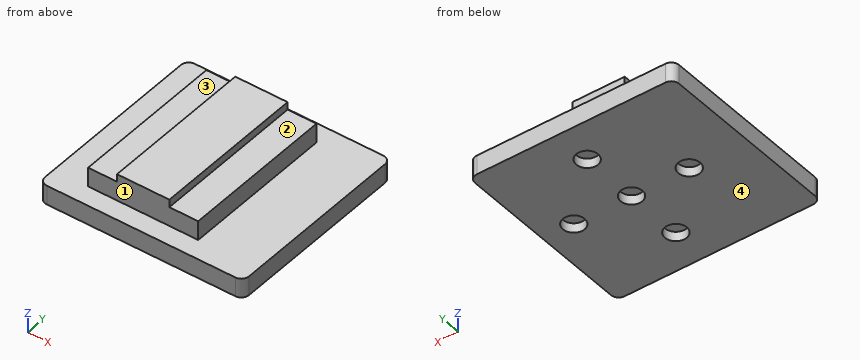
Autodesk Inventor part; units mm, degrees
ref_plane "YZ Plane" through (0, 0, 0) normal (1, 0, 0) x (0, 1, 0)
ref_plane "XZ Plane" through (0, 0, 0) normal (0, 1, 0) x (-1, 0, 0)
ref_plane "XY Plane" through (0, 0, 0) normal (0, 0, 1) x (1, 0, 0)
sketch "Sketch1" plane through (0, 0, 0) normal (0, 0, 1) x (1, 0, 0)
  line L0 (-24.5, 25) -> (24.5, 25)
  line L1 (26.5, 23) -> (26.5, -23)
  line L2 (24.5, -25) -> (-24.5, -25)
  line L3 (-26.5, -23) -> (-26.5, 23)
  arc A0 (-24.5, 25) -> (-26.5, 23) centre (-24.5, 23) ccw
  arc A1 (-26.5, -23) -> (-24.5, -25) centre (-24.5, -23) ccw
  arc A2 (24.5, -25) -> (26.5, -23) centre (24.5, -23) ccw
  arc A3 (26.5, 23) -> (24.5, 25) centre (24.5, 23) ccw
  point P0 (0, 0)
  point P1 (-26.5, 25)
  point P2 (26.5, -25)
  point P3 (26.5, 25)
  dimension "d0" = 53
  dimension "d2" = 2
  dimension "d3" = 25
  dimension "d4" = 50
  dimension "d5" = 26.5
extrude "base" add sketch "Sketch1" along normal blind 5
sketch "Sketch3" plane through (0, 0, 0) normal (0, 0, -1) x (-1, 0, 0)
  line L0 (26.5, 23) -> (26.5, -23)
  circle A0 centre (-3.5, 15) radius 2.825
  circle A1 centre (-18.5, 0) radius 2.825
  circle A2 centre (-3.5, 0) radius 2.825
  circle A3 centre (-3.5, -15) radius 2.825
  circle A4 centre (11.5, 0) radius 2.825
  point P0 (0, 0)
  dimension "d14" = 15
  dimension "d15" = 15
  dimension "d16" = 15
  dimension "d17" = 15
  dimension "d18" = 15
  dimension "d56" = 5.65
  dimension "d57" = 5.65
  dimension "d58" = 5.65
  dimension "d59" = 5.65
  dimension "d60" = 5.65
extrude "magnetExt" cut sketch "Sketch3" against normal blind 2.5
sketch "Sketch7" plane through (0, 0, 5) normal (0, 0, 1) x (1, 0, 0)
  line L0 (-17.6, 20) -> (11, 20)
  line L1 (11, 20) -> (11, -20)
  line L2 (11, -20) -> (-17.6, -20)
  line L3 (-17.6, -20) -> (-17.6, 20)
  line L4 (-26.5, 23) -> (-26.5, -23)
  point P0 (0, 0)
  dimension "d70" = 40
  dimension "d71" = 20
  dimension "d72" = 28.6
  dimension "d73" = 8.9
extrude "spacerOne" add sketch "Sketch7" along normal blind 5
sketch "Sketch8" plane through (0, 0, 10) normal (0, 0, 1) x (1, 0, 0)
  line L0 (-10.1, 20) -> (3.5, 20)
  line L1 (3.5, 20) -> (3.5, -20)
  line L2 (3.5, -20) -> (-10.1, -20)
  line L3 (-10.1, -20) -> (-10.1, 20)
  line L4 (-26.5, 23) -> (-26.5, -23)
  point P0 (0, 0)
  dimension "d76" = 40
  dimension "d77" = 20
  dimension "d78" = 13.6
  dimension "d79" = 30
extrude "sample" add sketch "Sketch8" along normal blind 2
equation "\"d56\" = d60"
equation "\"d57\" = d60"
equation "\"d58\" = d60"
equation "\"d59\" = d60"
equation "\"d1\" = d0"
properties part number "chamberInsertFlat"
Model file for the job. Use its own axes, mm. Face numbers are marked on the shaded views. A direction names the side the tool comes from. Round coordinates to 2 decimals unless told otherwise and drop trailing zeros. Loops run counter-clockwise (first coordinate to the right, second up) from the corner with the lowest first, then second, coordinate; pieces in that order, holes last.
1. Band-saw the part on C-C, the plane y = 0. List the corners of the cut face in (x, z) (3 decimals), and give its area (3 significant figures).
Check values:
outline: (-26.5, 0) - (-14.325, 0) - (-14.325, 2.5) - (-8.675, 2.5) - (-8.675, 0) - (0.675, 0) - (0.675, 2.5) - (6.325, 2.5) - (6.325, 0) - (15.675, 0) - (15.675, 2.5) - (21.325, 2.5) - (21.325, 0) - (26.5, 0) - (26.5, 5) - (11, 5) - (11, 10) - (3.5, 10) - (3.5, 12) - (-10.1, 12) - (-10.1, 10) - (-17.6, 10) - (-17.6, 5) - (-26.5, 5) - close
area: 393 mm2
2. Wall check: probe 1 along Y at (x, z) = (3.5, 0.95) (3 decimals); probe 2 along X at (y, z) = (-2.5, 1.25); probe 3 along Z at (x, y) = (22, 0). Give the ranges that are in metal, low to high.
Check values:
probe 1: y = -25 to -17.825, -12.175 to -2.825, 2.825 to 12.175, 17.825 to 25
probe 2: x = -26.5 to -12.82, -10.18 to 2.18, 4.82 to 17.18, 19.82 to 26.5
probe 3: z = 0 to 5
3. Band-saw the part on A-A, the plane y = -15. List the corners of the cut face in (x, z) (3 decimals).
Check values:
outline: (-26.5, 0) - (0.675, 0) - (0.675, 2.5) - (6.325, 2.5) - (6.325, 0) - (26.5, 0) - (26.5, 5) - (11, 5) - (11, 10) - (3.5, 10) - (3.5, 12) - (-10.1, 12) - (-10.1, 10) - (-17.6, 10) - (-17.6, 5) - (-26.5, 5) - close
4. Drop flat-ended pins along their axis: P1, Ø6, axis at x = -10.5, y = -13, coming from the +Z side; P2, Ø3, axis at x = -11.5, y = 0.5, coming from the -Z side; P3, Ø4, axis at x = 8.5, y = -1, coming from the +Z side; P4, Ø5, axis at x = 17.5, y = 3.5, coming from the +Z side. Give the stop position or say it passes through.
Check values:
P1: stops at z = 12
P2: stops at z = 2.5
P3: stops at z = 10
P4: stops at z = 5
5. Band-saw the part on D-D, the plane z = 10.75. List the corners of the cut face in (x, y), and give its area (3 significant figures).
Check values:
outline: (-10.1, -20) - (3.5, -20) - (3.5, 20) - (-10.1, 20) - close
area: 544 mm2
6. Tool access for the marked faces 1, 2, 3 and 4: list every direction of +Z, -Z, +X, -X, +Y, -Y with a clear straight run to the whole face (end or side of a thin tool).
Check values:
face 1: +Z, +X, -X, -Y
face 2: +Z, +X, +Y, -Y
face 3: +Z, -X, +Y, -Y
face 4: -Z, +X, -X, +Y, -Y
7. Band-saw the part on B-B, the plane x = 18.5. List the corners of the cut face in (y, z) (3 decimals), and give its area (3 significant figures).
Check values:
outline: (-25, 0) - (-2.825, 0) - (-2.825, 2.5) - (2.825, 2.5) - (2.825, 0) - (25, 0) - (25, 5) - (-25, 5) - close
area: 236 mm2
